Here's how the part is built. I have some questions about the finished solid (model axes, mm). A direction names the side the tool comes from. Round coordinates to 2 decimals unless told otherwise and drop trailing zeros. Write each loop counter-clockwise with the first axis right and the second up, starting at its lowest first coordinate (ties: lowest second). Pieces come first, ordered by that corner, then holes. Notation, with made-up numbers: (8.25, 36) - (35.25, 36) arc R13 ccw to (35.25, 47) - close; hole circle Ø11 at (33.25, -22.5). An arc over 180 degrees is marked (long way). Use one line per item in the form item = value. Start each with the question number.
1. If I drill on line 1 along Z through (x, y) = (0, -11); line 2 along Z through (x, y) = (9.5, -13.5); line 3 along X through (y, z) = (-5, 13), over which ranges is the centre line in solid material (lowest first)?
2. We'd pull the mould along X, two halves only. Please class faces 1 (the flat face through (6, -12, 20)), 2 (the cylindrical face through (13.1, -13.84, -18.31)), 3 (the cylindrical face through (13.11, -12.112, -10.956)), 4 (the flat face through (-14, 0, 20)): +X half, -X half, draft (parallel to the pull), parting line (faces both ways), or undercut.
3. I want a section at D-D, the plane x = 17. List the corners of the cut face in (y, z) for me, plus the area to 3 significant figures.
4. Will these pins go through, and if not, where does the flat tip stop? pin 1 (1.5 mm diameter, centred on x = 14.5, z = -13.5, fed in from -Y); pin 2 (1.5 mm diameter, centred on y = -12, z = -21, fed in from +X).
5. I want a section at C-C, the plane x = 0. List the corners of the cut face in (y, z) for me, plus the area to 3 significant figures.
6. I want a section at B-B, the plane y = 6. List the corners of the cut face in (x, z) for me.
7. I want a section at A-A, the plane z = 0. List the corners of the cut face in (x, y) for me.
8. Which directions (+Z, -Z, +X, -X, +Y, -Y) give clear straight access to the entire face, cutting with the end or side of a thin tool? Please do faces 5 (the flat face through (-13, -4, 13)), 6 (the cylindrical face through (13.1, 11.67, 22.48)), 7 (the flat face through (6, 0, -26)).
```python
from build123d import *

# Parameters (mm, degrees)
F1_DEPTH = 20
F2_R     = 14
F3_DEPTH = 40
F4_R     = 2.5
F5_DEPTH = 16
F6_R     = 2.5
F7_DEPTH = 14


with BuildPart() as f1:
    # F0 (on Front) → F1 (new body, symmetric)
    with BuildSketch(Plane.XZ):
        Polygon((20, -26), (20, 26), (-8, 26), (-20, 14), (-20, -14), (-8, -26), align=None)
    extrude(amount=F1_DEPTH, both=True)

    # F2 (on face) → F3 (cut)
    with BuildSketch(Plane.XZ.offset(20)):
        Circle(F2_R)
    extrude(amount=-F3_DEPTH, mode=Mode.SUBTRACT)

    # F4 (on face) → F5 (cut)
    with BuildSketch(Plane.XZ.offset(20)):
        with Locations((-13.435029, 13.435029)):
            Circle(F4_R)
        with Locations((13.435029, 13.435029)):
            Circle(F4_R)
        with Locations((-13.435029, -13.435029)):
            Circle(F4_R)
        with Locations((13.435029, -13.435029)):
            Circle(F4_R)
        with Locations((0, 19)):
            Circle(F4_R)
        with Locations((0, -19)):
            Circle(F4_R)
    extrude(amount=-F5_DEPTH, mode=Mode.SUBTRACT)

    # F6 (on face) → F7 (cut)
    with BuildSketch(Plane.YZ.offset(20)):
        with Locations((-12, 20)):
            Circle(F6_R)
        with Locations((12, 20)):
            Circle(F6_R)
        with Locations((12, -20)):
            Circle(F6_R)
        with Locations((-12, -20)):
            Circle(F6_R)
    extrude(amount=-F7_DEPTH, mode=Mode.SUBTRACT)


solid = f1.part
```
Model answer:
q1.line_1 = -26 to -21.5, -16.5 to -14, 14 to 16.5, 21.5 to 26
q1.line_2 = -26 to -22, -18 to -10.28, 10.28 to 18, 22 to 26
q1.line_3 = -20 to -15.9, -10.97 to -5.2, 5.2 to 10.97, 15.9 to 20
q2.face_1 = +X half
q2.face_2 = draft
q2.face_3 = undercut
q2.face_4 = -X half
q3.outline = (-20, -26) - (20, -26) - (20, 26) - (-20, 26) - close; hole circle Ø5 at (-12, -20); hole circle Ø5 at (-12, 20); hole circle Ø5 at (12, -20); hole circle Ø5 at (12, 20)
q3.area = 2,000 mm2
q4.pin_1 = -4
q4.pin_2 = 6
q5.outline = (-20, -26) - (20, -26) - (20, -14) - (-20, -14) - (-20, -16.5) - (-4, -16.5) - (-4, -21.5) - (-20, -21.5) - close; (-20, 14) - (20, 14) - (20, 26) - (-20, 26) - (-20, 21.5) - (-4, 21.5) - (-4, 16.5) - (-20, 16.5) - close
q5.area = 800 mm2
q6.outline = (-20, -14) - (-8, -26) - (20, -26) - (20, 26) - (-8, 26) - (-20, 14) - close; hole circle Ø28 at (0, 0)
q7.outline = (-20, -20) - (-14, -20) - (-14, 20) - (-20, 20) - close; (14, -20) - (20, -20) - (20, 20) - (14, 20) - close
q8.face_5 = -Y
q8.face_6 = +X
q8.face_7 = -Z, +X, -X, +Y, -Y
